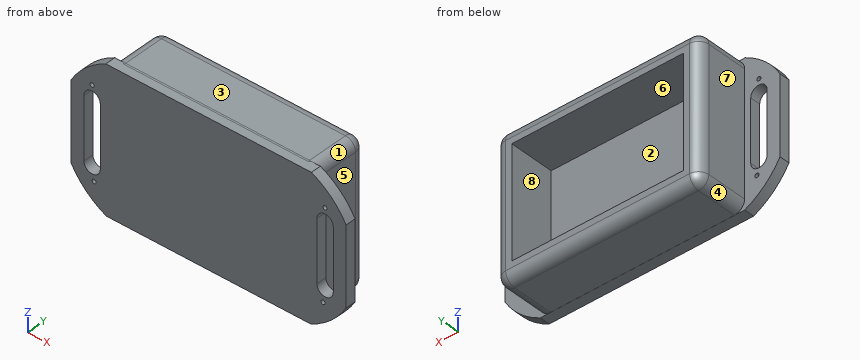
```python
from build123d import *

# Parameters (mm, degrees)
BOSS_EXTRUDE2_DEPTH = 15
FILLET2_R           = 2.5
SKETCH3_R           = 0.5
BOSS_EXTRUDE4_DEPTH = 2.5
SKETCH4_W           = 42.002754972
SKETCH4_H           = 27.001036704
CUT_EXTRUDE2_DEPTH  = 11


with BuildPart() as part:
    # Sketch1 → Boss-Extrude2 (new body)
    with BuildSketch(Plane(origin=(0, 0, 0), x_dir=(1, 0, 0), z_dir=(0, 1, 0))):
        with BuildLine():
            Line((-23.383883476, 16.616116524), (21.616116524, 16.616116524))
            ThreePointArc((21.616116524, 16.616116524), (23.383883476, 15.883883476), (24.116116524, 14.116116524))
            Line((24.116116524, 14.116116524), (24.116116524, -15.883883476))
            ThreePointArc((24.116116524, -15.883883476), (23.383883476, -17.651650429), (21.616116524, -18.383883476))
            Line((21.616116524, -18.383883476), (-23.383883476, -18.383883476))
            ThreePointArc((-23.383883476, -18.383883476), (-25.151650429, -17.651650429), (-25.883883476, -15.883883476))
            Line((-25.883883476, -15.883883476), (-25.883883476, 14.116116524))
            ThreePointArc((-25.883883476, 14.116116524), (-25.151650429, 15.883883476), (-23.383883476, 16.616116524))
        make_face()
    extrude(amount=BOSS_EXTRUDE2_DEPTH)

    # Fillet2
    fillet2_edges = [part.edges().sort_by_distance(p)[0] for p in [
        (-25.151650429, 15, 17.651650429),
        (-25.883883476, 0, 0.883883476),
        (-25.151650429, 0, -15.883883476),
        (-0.883883476, 15, 18.383883476),
        (23.383883476, 15, 17.651650429),
        (24.116116524, 15, 0.883883476),
        (23.383883476, 15, -15.883883476),
        (-0.883883476, 15, -16.616116524),
        (-25.151650429, 15, -15.883883476),
        (-25.883883476, 15, 0.883883476),
        (-0.883883476, 0, -16.616116524),
        (23.383883476, 0, -15.883883476),
        (24.116116524, 0, 0.883883476),
        (23.383883476, 0, 17.651650429),
        (-0.883883476, 0, 18.383883476),
        (-25.151650429, 0, 17.651650429),
    ]]
    fillet(fillet2_edges, radius=FILLET2_R)

    # Sketch3 → Boss-Extrude4 (add)
    with BuildSketch(Plane(origin=(0, 0, 0), x_dir=(1, 0, 0), z_dir=(0, 1, 0))):
        with BuildLine():
            Line((-25.883883476, 16.646945133), (24.116116524, 16.646945133))
            ThreePointArc((24.116116524, 16.646945133), (29.061870418, 13.334132498), (32.766116524, 8.674328862))
            Line((32.766116524, 8.674328862), (32.766116524, -10.453501419))
            ThreePointArc((32.766116524, -10.453501419), (29.124788001, -15.055056138), (24.271254893, -18.353054867))
            Line((24.271254893, -18.353054867), (-26.039021846, -18.353054867))
            ThreePointArc((-26.039021846, -18.353054867), (-30.892554954, -15.055056138), (-34.533883476, -10.453501419))
            Line((-34.533883476, -10.453501419), (-34.533883476, 8.674328862))
            ThreePointArc((-34.533883476, 8.674328862), (-30.829637371, 13.334132498), (-25.883883476, 16.646945133))
        make_face()
        with Locations(Location((-28.883883476, 10.158483361, 0), (0, 0, 270))):
            Circle(SKETCH3_R, mode=Mode.SUBTRACT)
        with Locations(Location((-29.383883476, -11.841516639, 0), (0, 0, 270))):
            Circle(SKETCH3_R, mode=Mode.SUBTRACT)
        with Locations(Location((27.616116524, -11.841516639, 0), (0, 0, 270))):
            Circle(SKETCH3_R, mode=Mode.SUBTRACT)
        with Locations(Location((27.116116524, 10.158483361, 0), (0, 0, 270))):
            Circle(SKETCH3_R, mode=Mode.SUBTRACT)
        with BuildLine():
            Line((29.616116524, 6.658483361), (29.616116524, -8.426250314))
            ThreePointArc((29.616116524, -8.426250314), (27.616116524, -10.426250314), (25.616116524, -8.426250314))
            Line((25.616116524, -8.426250314), (25.616116524, 6.658483361))
            ThreePointArc((25.616116524, 6.658483361), (27.616116524, 8.658483361), (29.616116524, 6.658483361))
        make_face(mode=Mode.SUBTRACT)
        with BuildLine():
            Line((-31.383883476, 6.658483361), (-31.383883476, -8.426250314))
            ThreePointArc((-31.383883476, -8.426250314), (-29.383883476, -10.426250314), (-27.383883476, -8.426250314))
            Line((-27.383883476, -8.426250314), (-27.383883476, 6.658483361))
            ThreePointArc((-27.383883476, 6.658483361), (-29.383883476, 8.658483361), (-31.383883476, 6.658483361))
        make_face(mode=Mode.SUBTRACT)
    extrude(amount=BOSS_EXTRUDE4_DEPTH)

    # Sketch4 → Cut-Extrude2 (cut)
    with BuildSketch(Plane(origin=(0, 15, 0), x_dir=(1, 0, 0), z_dir=(0, 1, 0))):
        with Locations((-0.88269634, -0.884055652)):
            Rectangle(SKETCH4_W, SKETCH4_H)
    extrude(amount=-CUT_EXTRUDE2_DEPTH, mode=Mode.SUBTRACT)


solid = part.part
```
Check sheet for the modelled part. Datum: model origin and axes. Units: mm. Face numbers are marked on the shaded views. A direction names the side the tool comes from. Round coordinates to 2 decimals unless told otherwise and drop trailing zeros. Order: outer loops, then holes, each group sorted by start corner. A loop starts at its lowest first (then second) coordinate and runs counter-clockwise, first axis right, second up. Notation, with made-up numbers: (26, 57) - (44, 57) arc R17 ccw to (44, 87) - close; hole circle Ø3 at (78.25, 52). An arc over 180 degrees is marked (long way). Answer as CSV lines item,"result". Start each with the question number.
1) Depth check by flat-ended pin: pin 1 (8 mm diameter, centred on x = -5, z = 1.5, fed in from +Y); pin 2 (2 mm diameter, centred on y = 4, z = -12, fed in from +X); pin 3 (3.5 mm diameter, centred on x = 6.5, y = 9, fed in from -Z). Enter the tip coordinate at first touch or a pass-through.
2) Section check B-B (z = -2). Record the cut outline in (x, y), then the cut area to 3 significant figures.
3) Scan lines: probe 1 along X at (y, z) = (1.5, -0.5); probe 2 along Z at (x, y) = (19, 6); probe 3 along X at (y, z) = (8.25, 2). Record each from-to range of solid material in increasing order.
4) Tool access check on the marked faces 1, 2, 3 and 4. Record the directions out of +Z, -Z, +X, -X, +Y, -Y that give a thin tool (end or side, any length) a straight path to the whole face; none if there is none.
5) Section check D-D (y = 14). Record the cut outline in (x, z).
6) Draft check along X on the marked faces 5, 6, 7 and 8. Enter one of: +X half, -X half, draft (parallel to the pull), parting line (faces both ways), or undercut.
7) Section check A-A (y = 6.75). Record the cut outline in (x, z), then the cut area to 3 significant figures.
Determined:
1,pin 1,"y = 4"
1,pin 2,"x = 24.12"
1,pin 3,"z = -16.62"
2,outline,"(-34.53, 0) - (-31.38, 0) - (-31.38, 2.5) - (-34.53, 2.5) - close; (-27.38, 0) - (25.62, 0) - (25.62, 2.5) - (24.12, 2.5) - (24.12, 12.5) arc R2.5 ccw to (21.62, 15) - (20.12, 15) - (20.12, 4) - (-21.88, 4) - (-21.88, 15) - (-23.38, 15) arc R2.5 ccw to (-25.88, 12.5) - (-25.88, 2.5) - (-27.38, 2.5) - close; (29.62, 0) - (32.77, 0) - (32.77, 2.5) - (29.62, 2.5) - close"
2,area,"309 mm^2"
3,probe 1,"-34.53 to -31.38, -27.38 to 25.62, 29.62 to 32.77"
3,probe 2,"-16.62 to -12.62, 14.38 to 18.38"
3,probe 3,"-25.88 to -21.88, 20.12 to 24.12"
4,face 1,"+Z, +X, +Y"
4,face 2,"+Y"
4,face 3,"+Z, +X, -X, +Y, -Y"
4,face 4,"-Z, -X, +Y"
5,outline,"(-25.38, -14.12) arc R2 ccw to (-23.38, -16.12) - (21.62, -16.12) arc R2 ccw to (23.62, -14.12) - (23.62, 15.88) arc R2 ccw to (21.62, 17.88) - (-23.38, 17.88) arc R2 ccw to (-25.38, 15.88) - close; hole (-21.88, -12.62) - (20.12, -12.62) - (20.12, 14.38) - (-21.88, 14.38) - close"
6,face 5,"+X half"
6,face 6,"undercut"
6,face 7,"-X half"
6,face 8,"undercut"
7,outline,"(-25.88, -14.12) arc R2.5 ccw to (-23.38, -16.62) - (21.62, -16.62) arc R2.5 ccw to (24.12, -14.12) - (24.12, 15.88) arc R2.5 ccw to (21.62, 18.38) - (-23.38, 18.38) arc R2.5 ccw to (-25.88, 15.88) - close; hole (-21.88, -12.62) - (20.12, -12.62) - (20.12, 14.38) - (-21.88, 14.38) - close"
7,area,"611 mm^2"
